Read the model definition and answer for the solid it produces. Units are mm, in the model's axes. A direction names the side the tool comes from. Give positions to 0.01 mm unless a question says otherwise; leave off trailing zeros. Order: outer loops, then holes, each group sorted by start corner. A loop starts at its lowest first (then second) coordinate and runs counter-clockwise, first axis right, second up. Notation, with made-up numbers: (11.25, 7.5) - (26.25, 7.5) arc R16 ccw to (26.25, 11.5) - close; hole circle Ø9 at (5, 34.5). An arc over 180 degrees is marked (long way). Write each question's results on one line, items separated by ' | '.
from build123d import *

# Parameters (mm, degrees)
SKETCH1_W           = 56
SKETCH1_H           = 56
BOSS_EXTRUDE1_DEPTH = 25
SKETCH2_W           = 53.2
SKETCH2_H           = 53.2
CUT_EXTRUDE1_DEPTH  = 22
SKETCH3_R           = 1.7
CUT_EXTRUDE2_DEPTH  = 1.4
SKETCH4_W           = 25.2
SKETCH4_H           = 27.2
CUT_EXTRUDE3_DEPTH  = 3
SKETCH5_W           = 4
SKETCH5_H           = 4
BOSS_EXTRUDE2_DEPTH = 3
SKETCH6_W           = 8
SKETCH6_H           = 8
BOSS_EXTRUDE3_DEPTH = 5
SKETCH7_R           = 2
CUT_EXTRUDE4_DEPTH  = 8
BOSS_EXTRUDE4_DEPTH = 3
FILLET1_R           = 1
CHAMFER1_SIZE       = 1.35
FILL_PATTERN1_DEPTH = 3


# Read off the part's stored shape, not the designer's step: Fill Pattern1
with BuildPart() as part:
    # Sketch1 → Boss-Extrude1 (new body)
    with BuildSketch(Plane(origin=(0, 0, 0), x_dir=(1, 0, 0), z_dir=(0, 1, 0))):
        Rectangle(SKETCH1_W, SKETCH1_H)
    extrude(amount=BOSS_EXTRUDE1_DEPTH)

    # Sketch2 → Cut-Extrude1 (cut)
    with BuildSketch(Plane(origin=(0, 25, 0), x_dir=(1, 0, 0), z_dir=(0, 1, 0))):
        Rectangle(SKETCH2_W, SKETCH2_H)
    extrude(amount=-CUT_EXTRUDE1_DEPTH, mode=Mode.SUBTRACT)

    # Sketch3 → Cut-Extrude2 (cut)
    with BuildSketch(Plane.XY.offset(28)):
        with Locations((0, 21.6)):
            Circle(SKETCH3_R)
    extrude(amount=-CUT_EXTRUDE2_DEPTH, mode=Mode.SUBTRACT)

    # Sketch4 → Cut-Extrude3 (cut)
    with BuildSketch(Plane.XZ):
        with Locations((0, 8.1)):
            Rectangle(SKETCH4_W, SKETCH4_H)
    extrude(amount=-CUT_EXTRUDE3_DEPTH, mode=Mode.SUBTRACT)

    # Sketch5 → Boss-Extrude2 (add)
    with BuildSketch(Plane.XZ):
        with Locations((-10.6, 19.7)):
            Rectangle(SKETCH5_W, SKETCH5_H)
        with Locations((10.6, 19.7)):
            Rectangle(SKETCH5_W, SKETCH5_H)
        with Locations((10.6, -3.5)):
            Rectangle(SKETCH5_W, SKETCH5_H)
        with Locations((-10.6, -3.5)):
            Rectangle(SKETCH5_W, SKETCH5_H)
    extrude(amount=-BOSS_EXTRUDE2_DEPTH)

    # Sketch6 → Boss-Extrude3 (add)
    with BuildSketch(Plane(origin=(0, 3, 0), x_dir=(1, 0, 0), z_dir=(0, 1, 0))):
        with Locations((16.6, -19.7)):
            Rectangle(SKETCH6_W, SKETCH6_H)
        with Locations((-16.6, -19.7)):
            Rectangle(SKETCH6_W, SKETCH6_H)
        Polygon((12.6, -0.5), (20.6, -0.5), (22.6, -0.5), (22.6, 9.5), (12.6, 9.5), (12.6, 7.5), align=None)
        Polygon((-12.6, -0.5), (-20.6, -0.5), (-22.6, -0.5), (-22.6, 9.5), (-12.6, 9.5), (-12.6, 7.5), align=None)
    extrude(amount=BOSS_EXTRUDE3_DEPTH)

    # Sketch7 → Cut-Extrude4 (cut)
    with BuildSketch(Plane(origin=(0, 8, 0), x_dir=(1, 0, 0), z_dir=(0, 1, 0))):
        with Locations(Location((16.6, -19.7, 0), (0, 0, 270))):
            Circle(SKETCH7_R)
        with Locations(Location((-16.6, -19.7, 0), (0, 0, 270))):
            Circle(SKETCH7_R)
        with Locations(Location((16.6, 3.5, 0), (0, 0, 270))):
            Circle(SKETCH7_R)
        with Locations(Location((-16.6, 3.5, 0), (0, 0, 270))):
            Circle(SKETCH7_R)
    extrude(amount=-CUT_EXTRUDE4_DEPTH, mode=Mode.SUBTRACT)

    # Sketch9 → Boss-Extrude4 (add)
    with BuildSketch(Plane(origin=(0, 8, 0), x_dir=(1, 0, 0), z_dir=(0, 1, 0))):
        Polygon((-22.6, -0.5), (-22.6, 9.5), (-12.6, 9.5), (-12.6, 7.5), (-20.6, 7.5), (-20.6, -0.5), align=None)
        Polygon((12.6, 9.5), (22.6, 9.5), (22.6, -0.5), (20.6, -0.5), (20.6, 7.5), (12.6, 7.5), align=None)
    extrude(amount=BOSS_EXTRUDE4_DEPTH)

    # Fillet1
    fillet1_edges = [part.edges().sort_by_distance(p)[0] for p in [
        (0, 0, 28),
        (-28, 0, 0),
        (0, 0, -28),
        (28, 0, 0),
        (28, 12.5, 28),
        (-28, 12.5, 28),
        (-28, 12.5, -28),
        (28, 12.5, -28),
    ]]
    fillet(fillet1_edges, radius=FILLET1_R)

    # Chamfer1
    chamfer1_edges = [part.edges().sort_by_distance(p)[0] for p in [
        (-1.7, 21.6, 28),
    ]]
    chamfer(chamfer1_edges, length=CHAMFER1_SIZE)

    # Fill Pattern1 outline → Fill Pattern1 (cut)
    with BuildSketch(Plane(origin=(0, 0, 0), x_dir=(1, 0, 0), z_dir=(0, 1, 0))):
        Polygon((22.516660498, 17), (24.248711306, 20), (22.516660498, 23), (19.052558883, 23), (17.320508076, 20), (19.052558883, 17), align=None)
        Polygon((8.660254038, 23), (5.196152423, 23), (3.464101615, 20), (5.196152423, 17), (8.660254038, 17), (10.392304845, 20), align=None)
        Polygon((-5.196152423, 23), (-8.660254038, 23), (-10.392304845, 20), (-8.660254038, 17), (-5.196152423, 17), (-3.464101615, 20), align=None)
        Polygon((-19.052558883, 23), (-22.516660498, 23), (-24.248711306, 20), (-22.516660498, 17), (-19.052558883, 17), (-17.320508076, 20), align=None)
        Polygon((1.732050808, 13), (3.464101615, 16), (1.732050808, 19), (-1.732050808, 19), (-3.464101615, 16), (-1.732050808, 13), align=None)
        Polygon((-12.124355653, 19), (-15.588457268, 19), (-17.320508076, 16), (-15.588457268, 13), (-12.124355653, 13), (-10.392304845, 16), align=None)
        Polygon((15.588457268, 19), (12.124355653, 19), (10.392304845, 16), (12.124355653, 13), (15.588457268, 13), (17.320508076, 16), align=None)
        Polygon((8.660254038, 9), (10.392304845, 12), (8.660254038, 15), (5.196152423, 15), (3.464101615, 12), (5.196152423, 9), align=None)
        Polygon((-5.196152423, 15), (-8.660254038, 15), (-10.392304845, 12), (-8.660254038, 9), (-5.196152423, 9), (-3.464101615, 12), align=None)
    extrude(amount=FILL_PATTERN1_DEPTH, mode=Mode.SUBTRACT)


solid = part.part
(1) Section B-B (z = -3.5) is taken. State how many separate pieces and enclosed holes the cut face has, plus the area to 3 significant figures.
Conclusion:
separate pieces: 4 | enclosed holes: 0 | area: 226 mm^2
(2) Section D-D (y = 21.6) is taken. Give the vertices of the cut face in (x, z), plus the area to 3 significant figures.
Conclusion:
outline: (-28, -27) arc R1 ccw to (-27, -28) - (27, -28) arc R1 ccw to (28, -27) - (28, 27) arc R1 ccw to (27, 28) - (3.05, 28) - (1.7, 26.65) - (1.7, 26.6) - (26.6, 26.6) - (26.6, -26.6) - (-26.6, -26.6) - (-26.6, 26.6) - (-1.7, 26.6) - (-1.7, 26.65) - (-3.05, 28) - (-27, 28) arc R1 ccw to (-28, 27) - close | area: 298 mm^2
(3) For faces 1 (the face through (-15, 8, -5)), 2 (the face through (2.6, 1.5, -14.5)), determine the directions among +Z, -Z, +X, -X, +Y, -Y from which every point of the face is accessible in a straight line to the end or side of a thin tool.
Conclusion:
face 1: +Y | face 2: +Y, -Y
(4) Section C-C (y = 11.75) is taken. Give the vertices of the cut face in (x, z), plus the area to 3 significant figures.
Conclusion:
outline: (-28, -27) arc R1 ccw to (-27, -28) - (27, -28) arc R1 ccw to (28, -27) - (28, 27) arc R1 ccw to (27, 28) - (-27, 28) arc R1 ccw to (-28, 27) - close; hole (-26.6, -26.6) - (26.6, -26.6) - (26.6, 26.6) - (-26.6, 26.6) - close | area: 305 mm^2
(5) The mould has two halves that part along Z. Classify faces 3 (the face through (4.32, 1.48, -10.52)), 4 (the face through (7, 1, -15)): pulls with the +Z half, pulls with the -Z half, needs draft (parallel to the pull), parting line crosses it, or undercut.
Conclusion:
face 3: undercut | face 4: undercut
(6) Consider probe 1 along X at (y, z) = (4, -3.5); probe 2 along Z at (x, y) = (-21, 5.25); probe 3 along X at (y, z) = (4.5, 19.7). Determine where each line is inside the solid, lowest interval first. Write a range as [from, to].
Conclusion:
probe 1: [-28, -26.6], [-22.6, -18.6], [-14.6, -12.6], [12.6, 14.6], [18.6, 22.6], [26.6, 28] | probe 2: [-28, -26.6], [-9.5, 0.5], [26.6, 28] | probe 3: [-28, -26.6], [-20.6, -18.6], [-14.6, -12.6], [12.6, 14.6], [18.6, 20.6], [26.6, 28]
(7) Section A-A (x = 0) is taken. Give the vertices of the cut face in (y, z), plus the area to 3 significant figures.
Conclusion:
outline: (0, -27) arc R1 ccw to (1, -28) - (25, -28) - (25, -26.6) - (3, -26.6) - (3, -19) - (0, -19) - close; (0, -13) - (3, -13) - (3, -5.5) - (0, -5.5) - close; (0, 21.7) - (3, 21.7) - (3, 26.6) - (19.9, 26.6) - (19.9, 26.65) - (18.55, 28) - (1, 28) arc R1 ccw to (0, 27) - close; (23.3, 26.6) - (25, 26.6) - (25, 28) - (24.65, 28) - (23.3, 26.65) - close | area: 123 mm^2
(8) Each of these flat-tipped pins is pushed along its axis until it touches: pin 1 (4.5 mm diameter, centred on x = 16.6, z = 19.7, fed in from +Y); pin 2 (4 mm diameter, centred on x = 0, y = 21.6, fed in from +Z); pin 3 (8 mm diameter, centred on x = 5, z = -20.5, fed in from +Y); pin 4 (5 mm diameter, centred on x = 16.6, z = -3.5, fed in from -Y). Where does it stop, or does it pass through?
Conclusion:
pin 1: y = 8 | pin 2: z = 26.95 | pin 3: y = 3 | pin 4: y = 0
